Could you check a few things on this drawing? It's one solid part, dimensions in mm from its lowest x, y, z. A direction names the side the tool comes from. Round coordinates to 2 decimals unless told otherwise and drop trailing zeros. Write each loop counter-clockwise with the first axis right and the second up, starting at its lowest first coordinate (ties: lowest second). Pieces come first, ordered by that corner, then holes. Notation, with made-up numbers: (14, 7.5) - (71, 7.5) arc R25 ccw to (71, 22.5) - close; hole circle Ø6 at (88, 51). An arc over 180 degrees is marked (long way). Use one line per item in the form item = value. Start each with the question number.
1. I want a section at C-C, the plane z = 88.9. List the corners of the cut face in (x, y) for me.
2. I want a section at A-A, the plane x = 17. List the corners of the cut face in (y, z) for me.
3. I want a section at D-D, the plane y = 25.4. List the corners of the cut face in (x, z) for me, plus the area to 3 significant figures.
4. If I drill on line 1 along X through (y, z) = (20, 33); line 2 along X through (y, z) = (3.2, 88.9); line 3 along X through (y, z) = (1.45, 88.9), over which ranges is the centre line in solid material (lowest first)?
5. I want a section at B-B, the plane x = 47. List the corners of the cut face in (y, z) for me, plus the area to 3 significant figures.
6. Will these pins go through, and if not, where does the flat tip stop? pin 1 (2 mm diameter, centred on y = 2, z = 45, fed in from -X) (3 decimals); pin 2 (8 mm diameter, centred on x = 83, z = 40, fed in from -Y); pin 3 (3 mm diameter, centred on y = 2.5, z = 51, fed in from +X); pin 4 (6 mm diameter, centred on x = 66.5, z = 19.5, fed in from +Y).
7. Which directions (+Z, -Z, +X, -X, +Y, -Y) give clear straight access to the entire face, cutting with the end or side of a thin tool? Please do the marked faces 5 and 6.
8. We'd pull the mould along X, two halves only. Please class the marked faces 1, 2, 3 and 4: +X half, -X half, draft (parallel to the pull), parting line (faces both ways), or undercut.
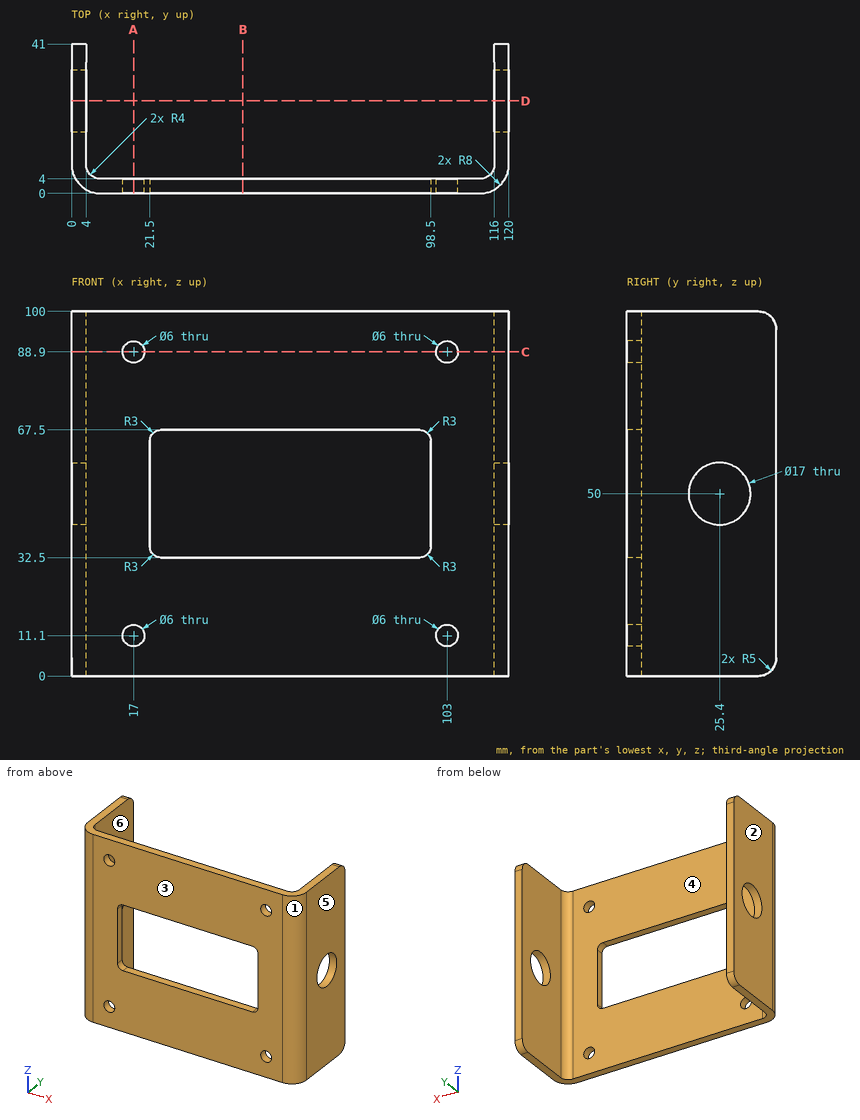
Model answer:
q1.outline = (0, 8) arc R8 ccw to (8, 0) - (14, 0) - (14, 4) - (8, 4) arc R4 cw to (4, 8) - (4, 41) - (0, 41) - close; (20, 0) - (100, 0) - (100, 4) - (20, 4) - close; (106, 0) - (112, 0) arc R8 ccw to (120, 8) - (120, 41) - (116, 41) - (116, 8) arc R4 cw to (112, 4) - (106, 4) - close
q2.outline = (0, 0) - (4, 0) - (4, 8.1) - (0, 8.1) - close; (0, 14.1) - (4, 14.1) - (4, 85.9) - (0, 85.9) - close; (0, 91.9) - (4, 91.9) - (4, 100) - (0, 100) - close
q3.outline = (0, 0) - (4, 0) - (4, 41.5) - (0, 41.5) - close; (0, 58.5) - (4, 58.5) - (4, 100) - (0, 100) - close; (116, 0) - (120, 0) - (120, 41.5) - (116, 41.5) - close; (116, 58.5) - (120, 58.5) - (120, 100) - (116, 100) - close
q3.area = 664 mm2
q4.line_1 = 0 to 4, 116 to 120
q4.line_2 = 1.6 to 14, 20 to 100, 106 to 118.4
q4.line_3 = 3.41 to 14, 20 to 100, 106 to 116.59
q5.outline = (0, 0) - (4, 0) - (4, 32.5) - (0, 32.5) - close; (0, 67.5) - (4, 67.5) - (4, 100) - (0, 100) - close
q5.area = 260 mm2
q6.pin_1 = 1.755
q6.pin_2 = through
q6.pin_3 = 118.93
q6.pin_4 = 4
q7.face_5 = +Z, -Z, +X, +Y, -Y
q7.face_6 = +Z, -Z, +Y
q8.face_1 = +X half
q8.face_2 = -X half
q8.face_3 = draft
q8.face_4 = undercut
